Here's how the part is built. I have some questions about the finished solid (model axes, mm). Give positions to 0.01 mm unless a question says otherwise; leave off trailing zeros. Write each loop counter-clockwise with the first axis right and the second up, starting at its lowest first coordinate (ties: lowest second). Pieces come first, ordered by that corner, then holes. Notation, with made-up numbers: M -37.5,44 L -33.5,44 A20 cw -33.5,75 Z; hole C 14.5,4 d10. An arc over 180 degrees is marked long. Answer as CSV lines item,"result". Start each with the question number.
Q1. Thinking about a two-plate mould opening in Z: for faces 1 (the flat face through (-2.03, 2.8, 1.65)), 2 (the cylindrical face through (-3.493, -0.631, 2.003)), 3 (the flat face through (0, 2, 0)), 4 (the flat face through (-2, 0, -3.25)), which applies, +Z half, -Z half, draft (parallel to the pull), parting line (faces both ways), or undercut?
Q2. If I drill on line 1 along Y through (x, z) = (-3.6, 0); line 2 along Y through (x, z) = (-0.5, 0); line 3 along Z through (x, y) = (-3.05, -1.5), over which ranges is the centre line in solid material (lowest first)?
Q3. Suppose I cut it at B-B (y = 0). Write out the boundary of the cut face in (x, z), then the cut area to 3 significant figures.
Q4. Suppose I cut it at A-A (z = 0). Write out the boundary of the cut face in (x, y), then the cut area to 3 significant figures.
Q5. Suppose I cut it at D-D (z = -1.75). Write out the boundary of the cut face in (x, y), then the cut area to 3 significant figures.
Q6. For pin 1 (1.5 mm diameter, centred on x = -3.5, z = 2, fed in from -Y), with a flat end and sliding along its axis, tell me the tip position at first contact or that it passes through.
Q7. Suppose I cut it at C-C (x = -2). Write out the boundary of the cut face in (y, z), then the cut area to 3 significant figures.
```python
from build123d import *

# Parameters (mm, degrees)
SKETCH_2_OUTSIDE_W  = 11.514
SKETCH_2_OUTSIDE_H  = 11.514
CUT_EXTRUDE_1_DEPTH = 10


with BuildPart() as part:
    # 草图1 → 旋转1 (revolve)
    with BuildSketch(Plane.XY, mode=Mode.PRIVATE) as revolve_1_sk:
        Polygon((0, 1.4), (0, 3.65), (-4, 3.65), (-4, 2.1), (-3, 2.1), (-3, 1.4), align=None)
    revolve(revolve_1_sk.sketch.rotate(Axis((-9.405405405, 0, 0), (1, 0, 0)), 90), axis=Axis((-9.405405405, 0, 0), (1, 0, 0)))

    # 草图2 outside → 切除-拉伸1 (cut)
    with BuildSketch(Plane.ZY.offset(4)):
        Rectangle(SKETCH_2_OUTSIDE_W, SKETCH_2_OUTSIDE_H)
        Polygon((0, 3.75277675), (-3.25, 1.876388375), (-3.25, -1.876388375), (0, -3.75277675), (3.25, -1.876388375), (3.25, 1.876388375), align=None, mode=Mode.SUBTRACT)
    extrude(amount=-CUT_EXTRUDE_1_DEPTH, mode=Mode.SUBTRACT)


solid = part.part
```
Resolved:
1,face 1,"+Z half"
1,face 2,"undercut"
1,face 3,"draft"
1,face 4,"-Z half"
2,line 1,"-3.65 to -2.1, 2.1 to 3.65"
2,line 2,"-3.65 to -1.4, 1.4 to 3.65"
2,line 3,"-3.25 to -1.47, 1.47 to 3.25"
3,outline,"M -4,-3.25 L 0,-3.25 L 0,-1.4 L -3,-1.4 L -3,-2.1 L -4,-2.1 Z; M -4,2.1 L -3,2.1 L -3,1.4 L 0,1.4 L 0,3.25 L -4,3.25 Z"
3,area,"13.4 mm^2"
4,outline,"M -4,-3.65 L 0,-3.65 L 0,-1.4 L -3,-1.4 L -3,-2.1 L -4,-2.1 Z; M -4,2.1 L -3,2.1 L -3,1.4 L 0,1.4 L 0,3.65 L -4,3.65 Z"
4,area,"16.6 mm^2"
5,outline,"M -4,-2.74 L 0,-2.74 L 0,2.74 L -4,2.74 L -4,1.16 L -3,1.16 L -3,-1.16 L -4,-1.16 Z"
5,area,"19.6 mm^2"
6,pin 1,"y = -3.03"
7,outline,"M -3.65,-0.19 L -1.98,-3.06 A3.65 ccw -1.66,-3.25 L 1.66,-3.25 A3.65 ccw 1.98,-3.06 L 3.65,-0.19 A3.65 ccw 3.65,0.19 L 1.98,3.06 A3.65 ccw 1.66,3.25 L -1.66,3.25 A3.65 ccw -1.98,3.06 L -3.65,0.19 A3.65 ccw Z; hole C 0,0 d2.8"
7,area,"30.3 mm^2"
